Source: CAD feature listing. Evaluate the final solid. Frame: model axes, mm. A direction names the side the tool comes from. Round coordinates to 2 decimals unless told otherwise and drop trailing zeros. Order: outer loops, then holes, each group sorted by start corner. A loop starts at its lowest first (then second) coordinate and runs counter-clockwise, first axis right, second up. Notation, with made-up numbers: M 67.25,29 L 85.25,29 A6 cw 85.25,33 Z; hole C 6.25,-36 d7. An arc over 180 degrees is marked long. Use CSV: the item, a comma, the result in double quotes. Start each with the question number.
```python
from build123d import *

# Parameters (mm, degrees)
SKETCH1_R           = 13.5
BOSS_EXTRUDE1_DEPTH = 25
SKETCH2_R           = 2.5
BOSS_EXTRUDE2_DEPTH = 25
FILLET1_R           = 3
CHAMFER1_SIZE       = 5
SKETCH3_R           = 1.6
BOSS_EXTRUDE3_DEPTH = 2
SKETCH4_R           = 4
CUT_EXTRUDE1_DEPTH  = 2


with BuildPart() as part:
    # Sketch1 → Boss-Extrude1 (new body)
    with BuildSketch(Plane.XY):
        Circle(SKETCH1_R)
    extrude(amount=BOSS_EXTRUDE1_DEPTH)

    # Sketch2 → Boss-Extrude2 (add)
    with BuildSketch(Plane.XY.offset(25)):
        Circle(SKETCH2_R)
    extrude(amount=BOSS_EXTRUDE2_DEPTH)

    # Fillet1
    fillet1_edges = [part.edges().sort_by_distance(p)[0] for p in [
        (-13.5, 0, 0),
    ]]
    fillet(fillet1_edges, radius=FILLET1_R)

    # Chamfer1
    chamfer1_edges = [part.edges().sort_by_distance(p)[0] for p in [
        (-13.5, 0, 25),
    ]]
    chamfer(chamfer1_edges, length=CHAMFER1_SIZE)

    # Sketch3 → Boss-Extrude3 (add)
    with BuildSketch(Plane(origin=(0, 0, 0), x_dir=(-1, 0, 0), z_dir=(0, 0, -1))):
        with BuildLine():
            Line((-3.5, -7.5), (-3.5, -16))
            ThreePointArc((-3.5, -16), (-2.5, -18.645751311), (0, -19.968626967))
            ThreePointArc((0, -19.968626967), (2.5, -18.645751311), (3.5, -16))
            Line((3.5, -16), (3.5, -7.5))
            ThreePointArc((3.5, -7.5), (4.671572875, -4.671572875), (7.5, -3.5))
            Line((7.5, -3.5), (16, -3.5))
            ThreePointArc((16, -3.5), (18.645751311, -2.5), (19.968626967, 0))
            ThreePointArc((19.968626967, 0), (18.645751311, 2.5), (16, 3.5))
            Line((16, 3.5), (7.5, 3.5))
            ThreePointArc((7.5, 3.5), (4.671572875, 4.671572875), (3.5, 7.5))
            Line((3.5, 7.5), (3.5, 16))
            ThreePointArc((3.5, 16), (2.5, 18.645751311), (0, 19.968626967))
            ThreePointArc((0, 19.968626967), (-2.5, 18.645751311), (-3.5, 16))
            Line((-3.5, 16), (-3.5, 7.5))
            ThreePointArc((-3.5, 7.5), (-4.671572875, 4.671572875), (-7.5, 3.5))
            Line((-7.5, 3.5), (-16, 3.5))
            ThreePointArc((-16, 3.5), (-18.645751311, 2.5), (-19.968626967, 0))
            ThreePointArc((-19.968626967, 0), (-18.645751311, -2.5), (-16, -3.5))
            Line((-16, -3.5), (-7.5, -3.5))
            ThreePointArc((-7.5, -3.5), (-4.671572875, -4.671572875), (-3.5, -7.5))
        make_face()
        with Locations((-16.5, 0)):
            Circle(SKETCH3_R, mode=Mode.SUBTRACT)
        with Locations((0, 16.5)):
            Circle(SKETCH3_R, mode=Mode.SUBTRACT)
        with Locations((16.5, 0)):
            Circle(SKETCH3_R, mode=Mode.SUBTRACT)
        with Locations((0, -16.5)):
            Circle(SKETCH3_R, mode=Mode.SUBTRACT)
    extrude(amount=BOSS_EXTRUDE3_DEPTH)

    # Sketch4 → Cut-Extrude1 (cut)
    with BuildSketch(Plane(origin=(0, 0, -2), x_dir=(-1, 0, 0), z_dir=(0, 0, -1))):
        Circle(SKETCH4_R)
    extrude(amount=-CUT_EXTRUDE1_DEPTH, mode=Mode.SUBTRACT)


solid = part.part
```
(1) Reachability of faces 4 (the face through (-2.93, -13.18, 11.38)), 5 (the face through (-12, 3.5, -1)), 6 (the face through (6, 6, 0)), 7 (the face through (12, -3.5, -1)), 8 (the face through (-18.68, 2.47, -0.99)) from +Z, -Z, +X, -X, +Y, -Y: full face, straight path, thin tool, end or side. Return the list, or none.
(2) Section A-A on z = 45. Return loops of the section in (x, y), plus the area to 3 significant figures.
(3) Line query: line 1 along Z through (x, y) = (12, 3); line 2 along Z through (x, y) = (-12.5, 3); line 3 along Z through (x, y) = (18, -2). Output: solid intervals per line, ascending.
(4) Section B-B on z = 4. Return loops of the section in (x, y).
(5) Draft query along Y for faces 1 (the face through (-2.47, -18.68, -0.99)), 2 (the face through (-0.54, -2.44, 37.33)), 3 (the face through (0.208, 18.086, -0.986)). Return one class per face: pulls with the +Y half, pulls with the -Y half, needs draft (parallel to the pull), parting line crosses it, or undercut.
(6) Contact query for flat-ended pins moving along their axis: P1, Ø3, axis at x = 7.5, y = 6.5, coming from the -Z side; P2, Ø5, axis at x = 16.5, y = 0, coming from the +Z side; P3, Ø2, axis at x = -1, z = 21.5, coming from the +Y side; P4, Ø4, axis at x = 0, y = 16.5, coming from the -Z side. Output: stop coordinate, or through.
Results below:
1,face 4,"+Z"
1,face 5,"-Z, -X, +Y"
1,face 6,"-Z, +X, +Y"
1,face 7,"-Z, +X, -Y"
1,face 8,"+Z, -Z, -X, +Y"
2,outline,"C 0,0 d5"
2,area,"19.6 mm2"
3,line 1,"z = -2 to 0, 0.65 to 21.13"
3,line 2,"z = -2 to 0, 1.14 to 20.65"
3,line 3,"z = -2 to 0"
4,outline,"C 0,0 d27"
5,face 1,"pulls with the -Y half"
5,face 2,"parting line crosses it"
5,face 3,"undercut"
6,P1,"stops at z = 0"
6,P2,"stops at z = 0"
6,P3,"stops at y = 12.96"
6,P4,"stops at z = -2"
